Can you work these out from the model? Positions are in its coordinate system, mm. A direction names the side the tool comes from. Round coordinates to 2 decimals unless told otherwise and drop trailing zeros. Loops run counter-clockwise (first coordinate to the right, second up) from the corner with the lowest first, then second, coordinate; pieces in that order, holes last. Notation, with made-up numbers: M 28,33 L 63,33 A22 cw 63,43 Z; hole C 43,-19 d9. An arc over 180 degrees is marked long. Return JSON: item names as keys, results as strings.
```python
from build123d import *

# Parameters (mm, degrees)
F0_W        = 35
F0_H        = 30
F1_DEPTH    = 2
F2_W        = 4
F2_H        = 15
F3_DEPTH    = 5
F4_R        = 1
F5_DEPTH    = 25
F6_T1_DEPTH = 25.8639610307
F7_W        = 4
F7_H        = 15
F8_DEPTH    = 25


# Not quite as in the source:
# - a fillet or chamfer that OpenCascade refuses, or shapes differently, is made with other operations: its cross-section is extruded or revolved along the edge and cut away or added


with BuildPart() as f1:
    # F0 (on Top) → F1 (new body)
    with BuildSketch(Plane.XY):
        with Locations((-17.5, 0)):
            Rectangle(F0_W, F0_H)
    extrude(amount=F1_DEPTH)

    # F2 (on face) → F3 (join)
    with BuildSketch(Plane.XY.offset(2)):
        with Locations((-2, 7.5)):
            Rectangle(F2_W, F2_H)
    extrude(amount=F3_DEPTH)

    # F4 (on face) → F5 (cut)
    with BuildSketch(Plane.XZ):
        with Locations((-1.9937221408, 4.9999934314)):
            Circle(F4_R)
    extrude(amount=-F5_DEPTH, mode=Mode.SUBTRACT)

    # F6: fillet of radius 2.1727922061 on 2 edges, made by hand

    # F6_s2 → F6_t1 (cut)
    with BuildSketch(Plane.XZ.offset(-20.4319805153)):
        with BuildLine():
            ThreePointArc((-1.8272077939, 7), (-3.3636038969, 6.3636038969), (-4, 4.8272077939))
            Line((-4, 4.8272077939), (-4, 7))
            Line((-4, 7), (-1.8272077939, 7))
        make_face()
        with BuildLine():
            ThreePointArc((0, 4.8272077939), (-0.6363961031, 6.3636038969), (-2.1727922061, 7))
            Line((-2.1727922061, 7), (0, 7))
            Line((0, 7), (0, 4.8272077939))
        make_face()
    extrude(amount=F6_T1_DEPTH, mode=Mode.SUBTRACT)

    # F7 (on face) → F8 (cut)
    with BuildSketch(Plane.XY.offset(2)):
        with Locations((-2, -7.5)):
            Rectangle(F7_W, F7_H)
    extrude(amount=-F8_DEPTH, mode=Mode.SUBTRACT)


solid = f1.part
```
Q1. Suppose I cut it at C-C, the plane x = -24.5. Please give me the cut outline in (y, z), plus the area to 3 significant figures.
Results:
{"outline": "M -15,0 L 15,0 L 15,2 L -15,2 Z", "area": "60.0 mm2"}
Q2. Suppose I cut it at B-B, the plane z = 1. Please give me the cut outline in (x, y), plus the area to 3 significant figures.
Results:
{"outline": "M -35,-15 L -4,-15 L -4,0 L 0,0 L 0,15 L -35,15 Z", "area": "990 mm2"}
Q3. I'm going to push flat-ended pins straight in: pin 1 Ø6 at (x, y) = (-15.5, 11.5) entering from +Z; pin 2 Ø1.2 at (x, z) = (-1.99, 5) entering from +Y; pin 3 Ø1.5 at (y, z) = (5.5, 4) entering from -X; pin 4 Ø2 at (y, z) = (-5, 1.5) entering from +X. Where does each tip first touch, or does it pass through?
Results:
{"pin 1": "stops at z = 2", "pin 2": "passes through", "pin 3": "stops at x = -4", "pin 4": "stops at x = -4"}
Q4. Suppose I cut it at D-D, the plane y = -1. Please give me the cut outline in (x, z), plus the area to 3 significant figures.
Results:
{"outline": "M -35,0 L -4,0 L -4,2 L -35,2 Z", "area": "62.0 mm2"}
Q5. Thinking about a two-plate mould opening in X: for faces 4 (the flat face through (-18, 0, 0)), 5 (the flat face through (0, 7, 2)), 6 (the flat face through (-4, 7, 3)), 7 (the cylindrical face through (-2, 7, 6)), which applies, pulls with the +X half, pulls with the -X half, needs draft (parallel to the pull), parting line crosses it, or undercut?
Results:
{"face 4": "needs draft", "face 5": "pulls with the +X half", "face 6": "pulls with the -X half", "face 7": "undercut"}
Q6. If I drill on line 1 along X through (y, z) = (-13.25, 0.5); line 2 along Z through (x, y) = (-14.5, -2.5); line 3 along Y through (x, z) = (-2.5, 6), over which ranges is the centre line in solid material (lowest first)?
Results:
{"line 1": "x = -35 to -4", "line 2": "z = 0 to 2", "line 3": "y = 0 to 15"}
Q7. On a 3-axis mill with a long thin cutter (end or side, diameter ignored), from which of +Z, -Z, +X, -X, +Y, -Y can I reach the whole of each face in a straight line? I mean faces 1 (the flat face through (-20, 0, 2)), 2 (the cylindrical face through (-0.561, 7.605, 6.285)), 3 (the flat face through (-2, 0, 3)). Say none if no direction works.
Results:
{"face 1": "+Z, -X, +Y, -Y", "face 2": "+Z, +X, +Y, -Y", "face 3": "+Z, -Z, +X, -Y"}
Q8. Suppose I cut it at A-A, the plane y = 6.5. Please give me the cut outline in (x, z).
Results:
{"outline": "M -35,0 L 0,0 L 0,4.83 A2.17 ccw -2,6.99 A2.17 ccw -4,4.83 L -4,2 L -35,2 Z; hole C -1.99,5 d2"}
